Design review of the part built by this model. Coordinates are the model's own, in mm. A direction names the side the tool comes from. Coordinates: 2 decimals unless noted, no trailing zeros. Write each loop counter-clockwise with the first axis right and the second up, starting at its lowest first coordinate (ties: lowest second). Pieces come first, ordered by that corner, then holes.
Q1. Take a section at A-A, the plane x = 19.5. Write out the cut boundary in (y, z), plus the area to 3 significant figures.
Q2. Take a section at C-C, the plane y = 60. Write out the cut boundary in (x, z), plus the area to 3 significant figures.
Q3. For faces 5 (the flat face through (10, 217.665, -39)), 6 (the flat face through (2.8, -32.1, -4.5)), 7 (the flat face through (8, 220.665, -39)), list the 3-axis set-ups (+Z, -Z, +X, -X, +Y, -Y) from which the entire face can be reached by the end or side of a thin tool; tool diameter is ignored.
Q4. The part is to be moulded in two halves that separate along Z. For faces 1 (the flat face through (1, 85, 0)), 2 (the flat face through (2.7, -32.1, -3)), 3 (the flat face through (3, 83, -39)), 4 (the flat face through (1, 85, -80)), say which applies: released by +Z, released by -Z, zero draft, split by the parting line, or undercut.
Q5. For L1, parallel to Y at x = 9.5, z = -34; L2, parallel to Y at x = 56, z = -71.5; L3, parallel to X at y = 44.5, z = -19.5, list the stretches that pass through material, from the lowest coordinate up.
Q6. Take a section at D-D, the plane x = 77.5. Write out the cut boundary in (y, z).
Q7. Take a section at B-B, the plane y = -17.5. Write out the cut boundary in (x, z).
Q8. For pin 1 Ø3 at (x, z) = (72.5, -32) entering from +Y (3 decimals); pin 2 Ø1.5 at (y, z) = (218.5, -25) entering from +X; pin 3 Ø1.2 at (y, z) = (-19, -3.5) entering from +X, all flat-tipped, find the tip position at first contact; note any pin that passes through.
from build123d import *

# Parameters (mm, degrees)
BOSS_EXTRUDE1_DEPTH = 80
SKETCH2_W           = 1.5
SKETCH2_H           = 50
CUT_EXTRUDE1_DEPTH  = 1.5
CUT_EXTRUDE3_DEPTH  = 1.5


with BuildPart() as part:
    # Sketch1 → Boss-Extrude1 (new body)
    with BuildSketch(Plane.XY):
        Polygon((0, 220.664977974), (0, -51.835022026), (85.3, -51.835022026), (85.3, -48.835022026), (3, -48.835022026), (3, 217.664977974), (16.5, 217.664977974), (16.5, 220.664977974), align=None)
    extrude(amount=-BOSS_EXTRUDE1_DEPTH)

    # Sketch2 → Cut-Extrude1 (cut)
    with BuildSketch(Plane(origin=(3, 0, 0), x_dir=(0, 0, -1), z_dir=(1, 0, 0))):
        with Locations((3.75, -23.835022026)):
            Rectangle(SKETCH2_W, SKETCH2_H)
    extrude(amount=-CUT_EXTRUDE1_DEPTH, mode=Mode.SUBTRACT)

    # Sketch3 → Cut-Extrude3 (cut)
    with BuildSketch(Plane(origin=(0, -48.835022026, 0), x_dir=(1, 0, 0), z_dir=(0, 1, 0))):
        Polygon((2.83445579, 3), (24.563412283, 3), (24.563412283, 4.5), (1.5, 4.5), (1.5, 3), align=None)
    extrude(amount=-CUT_EXTRUDE3_DEPTH, mode=Mode.SUBTRACT)


solid = part.part
Responses:
1. outline: (-51.84, -80) - (-48.84, -80) - (-48.84, -4.5) - (-50.34, -4.5) - (-50.34, -3) - (-48.84, -3) - (-48.84, 0) - (-51.84, 0) - close
1. area: 238 mm2
2. outline: (0, -80) - (3, -80) - (3, 0) - (0, 0) - close
2. area: 240 mm2
3. face 5: +Z, -Z, +X
3. face 6: none
3. face 7: +Z, -Z, +X, -X, +Y
4. face 1: released by +Z
4. face 2: undercut
4. face 3: zero draft
4. face 4: released by -Z
5. L1: y = -51.84 to -48.84, 217.66 to 220.66
5. L2: y = -51.84 to -48.84
5. L3: x = 0 to 3
6. outline: (-51.84, -80) - (-48.84, -80) - (-48.84, 0) - (-51.84, 0) - close
7. outline: (0, -80) - (3, -80) - (3, -4.5) - (1.5, -4.5) - (1.5, -3) - (3, -3) - (3, 0) - (0, 0) - close
8. pin 1: stops at y = -48.835
8. pin 2: stops at x = 16.5
8. pin 3: stops at x = 3
